Could you check a few things on this drawing? It's one solid part, dimensions in mm from its lowest x, y, z. A direction names the side the tool comes from. Give positions to 0.01 mm unless a question says otherwise; leave off trailing zeros. Loops run counter-clockwise (first coordinate to the right, second up) from the corner with the lowest first, then second, coordinate; pieces in that order, holes last. Notation, with made-up numbers: (-23, 28) - (-16, 28) arc R13 cw to (-16, 40) - close; hole circle Ø5 at (38.5, 8.25). An arc over 180 degrees is marked (long way). Return JSON: item names as keys, results as strings. Group by question number.
(1) On a 3-axis mill with a long thin cutter (end or side, diameter ignored), from which of +Z, -Z, +X, -X, +Y, -Y can I reach the whole of each face in a straight line? I mean the marked faces 1 and 2. Say none if no direction works.
(2) If we mould it in two halves opening along Z, with no side actions, what happens to the marked faces 3, 4, 5 and 6? For each: released by +Z, released by -Z, zero draft, split by the parting line, or undercut.
(3) I need wall thicknesses on probe 1 along Z at (x, y) = (7.5, 4.15); probe 2 along Y at (x, z) = (14, 11) (3 decimals); probe 3 along Y at (x, z) = (8.5, 5.75) (3 decimals). Which ranges of each line are inside material? Lowest first, please. Write a range as [from, to].
(4) If we section it at C-C (y = 4.1): Please give me the cut outline in (x, z), then the cut area to 3 significant figures.
(5) If we section it at B-B (z = 3): State how many separate pieces and enclosed holes the cut face has, then the cut area to 3 significant figures.
(6) If we section it at A-A (x = 7.5): Please give me the cut outline in (y, z) (3 decimals).
(7) For P1, Ø0.6, axis at y = 2.5, z = 2, coming from the -X side; P2, Ø4, axis at x = 5.5, z = 5.5, coming from the -Y side; P3, Ø1.6, axis at x = 14.5, y = 1.5, coming from the -Z side, each with a flat end and sliding along its axis, tell me the tip position at first contact or that it passes through.
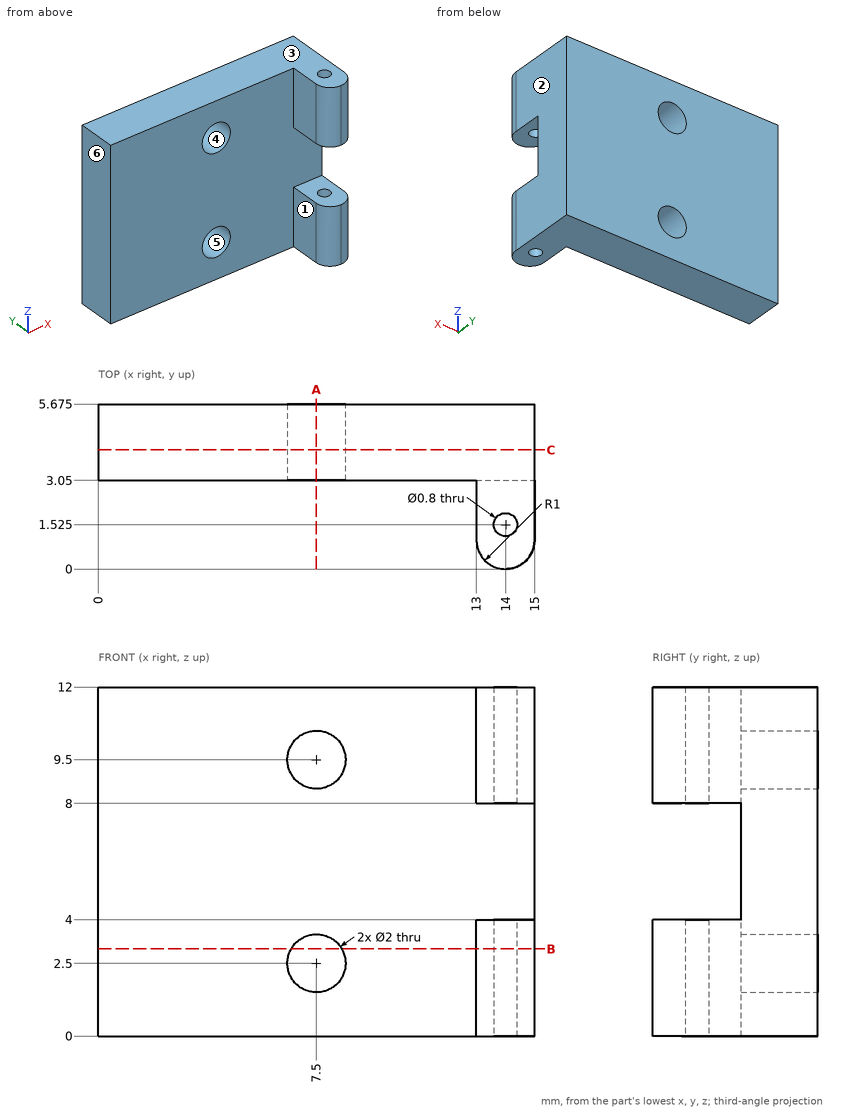
Values:
{
 "1": {"face 1": "+Z, -Z, -X, -Y", "face 2": "+Z, -Z, +X, +Y, -Y"},
 "2": {"face 3": "released by +Z", "face 4": "undercut", "face 5": "undercut", "face 6": "zero draft"},
 "3": {"probe 1": "[0, 1.5], [3.5, 8.5], [10.5, 12]", "probe 2": "[0, 1.125], [1.925, 5.675]", "probe 3": "[3.05, 5.675]"},
 "4": {"outline": "(0, 0) - (15, 0) - (15, 12) - (0, 12) - close; hole circle Ø2 at (7.5, 2.5); hole circle Ø2 at (7.5, 9.5)", "area": "174 mm2"},
 "5": {"separate pieces": "2", "enclosed holes": "1", "area": "40.0 mm2"},
 "6": {"outline": "(3.05, 0) - (5.675, 0) - (5.675, 1.5) - (3.05, 1.5) - close; (3.05, 3.5) - (5.675, 3.5) - (5.675, 8.5) - (3.05, 8.5) - close; (3.05, 10.5) - (5.675, 10.5) - (5.675, 12) - (3.05, 12) - close"},
 "7": {"P1": "x = 13", "P2": "y = 3.05", "P3": "z = 0"}
}
